```python
from build123d import *

# Parameters (mm, degrees)
SKETCH1_W           = 48
SKETCH1_H           = 5.175
SKETCH1_H_2         = 3
SKETCH1_H_3         = 3.35
BOSS_EXTRUDE1_DEPTH = 2
SKETCH1_3_W         = 48
SKETCH1_3_H         = 3
BOSS_EXTRUDE2_DEPTH = 8.5
CUT_EXTRUDE1_DEPTH  = 27.740991474
CHAMFER1_SIZE       = 0.5


with BuildPart() as part:
    # Sketch1 → Boss-Extrude1 (new body)
    with BuildSketch(Plane.XY):
        with Locations((0, 2.5875)):
            Rectangle(SKETCH1_W, SKETCH1_H)
        with Locations((0, 6.675)):
            Rectangle(SKETCH1_W, SKETCH1_H_2)
        with Locations((0, 9.85)):
            Rectangle(SKETCH1_W, SKETCH1_H_3)
    extrude(amount=BOSS_EXTRUDE1_DEPTH)

    # Sketch1_3 → Boss-Extrude2 (add)
    with BuildSketch(Plane.XY):
        with Locations((0, 6.675)):
            Rectangle(SKETCH1_3_W, SKETCH1_3_H)
    extrude(amount=BOSS_EXTRUDE2_DEPTH)

    # Sketch2 → Cut-Extrude1 (cut, through all)
    with BuildSketch(Plane(origin=(0, 8.175, 0), x_dir=(1, 0, 0), z_dir=(0, 1, 0))):
        with BuildLine():
            Line((-15, -6), (-15, -8.5))
            Line((-15, -8.5), (-10, -8.5))
            Line((-10, -8.5), (-10, -6))
            ThreePointArc((-10, -6), (-12.5, -3.5), (-15, -6))
        make_face()
        with BuildLine():
            Line((10, -8.5), (10, -6))
            ThreePointArc((10, -6), (12.5, -3.5), (15, -6))
            Line((15, -6), (15, -8.5))
            Line((15, -8.5), (10, -8.5))
        make_face()
    extrude(amount=-CUT_EXTRUDE1_DEPTH, mode=Mode.SUBTRACT)

    # Chamfer1
    chamfer1_edges = [part.edges().sort_by_distance(p)[0] for p in [
        (-24, 8.175, 5.25),
        (-24, 5.175, 5.25),
        (24, 5.175, 5.25),
        (24, 8.175, 5.25),
        (-19.5, 8.175, 8.5),
        (-19.5, 5.175, 8.5),
        (0, 5.175, 8.5),
        (19.5, 5.175, 8.5),
        (0, 8.175, 8.5),
        (19.5, 8.175, 8.5),
        (-15, 6.675, 8.5),
        (-10, 6.675, 8.5),
        (15, 6.675, 8.5),
        (10, 6.675, 8.5),
    ]]
    chamfer(chamfer1_edges, length=CHAMFER1_SIZE)


solid = part.part
```
Can you work these out from the model? Positions are in its coordinate system, mm. A direction names the side the tool comes from. Round coordinates to 2 decimals unless told otherwise and drop trailing zeros. Loops run counter-clockwise (first coordinate to the right, second up) from the corner with the lowest first, then second, coordinate; pieces in that order, holes last. Notation, with made-up numbers: M 43,8.5 L 56,8.5 A36 cw 56,46.5 Z; hole C 34,53.25 d9. An arc over 180 degrees is marked long. Answer as a JSON object with one key per item and string values. Group by question number.
Q1. Please list where these lines run through material, in increasing order: L1, parallel to X at y = 6, z = 7.5; L2, parallel to Y at x = 8, z = 5.75 (3 decimals); L3, parallel to Z at x = -2.5, y = 2.5.
Q2. Imagine slicing it at A-A, the plane x = -11. Please give me the cut outline in (y, z) (3 decimals).
Q3. On a 3-axis mill with a long thin cutter (end or side, diameter ignored), from which of +Z, -Z, +X, -X, +Y, -Y can I reach the whole of each face in a straight line? I mean faces 5 (the flat face through (0, 5.175, 5)), 6 (the flat face through (10, 7, 7)), 7 (the flat face through (0, 8.175, 5)). Say none if no direction works.
Q4. Imagine slicing it at C-C, the plane x = 16. Please give me the cut outline in (y, z) (3 decimals), then the cut area to 3 significant figures.
Q5. Will these pins go through, and if not, where does the flat tip stop? pin 1 (1.2 mm diameter, centred on x = -2.5, y = 9, fed in from +Z); pin 2 (3 mm diameter, centred on x = -2, z = 5, fed in from +Y) (3 decimals); pin 3 (1.5 mm diameter, centred on x = -8.5, y = 8.5, fed in from +Z) (3 decimals).
Q6. Imagine slicing it at B-B, the plane z = 5. Please give me the cut outline in (x, y) (3 decimals), then the cut area to 3 significant figures.
Q7. Imagine slicing it at D-D, the plane y = 1. Please give me the cut outline in (x, z).
Q8. We'd pull the mould along X, two halves only. Please class faces 1 (the cylindrical face through (-12.4, 6.7, 3.5)), 2 (the flat face through (0, 2, 2)), 3 (the flat face through (-15, 7, 7)), 4 (the flat face through (24, 6, 2)): +X half, -X half, draft (parallel to the pull), parting line (faces both ways), or undercut.
Findings:
{
 "1": {"L1": "x = -24 to -15, -10 to 10, 15 to 24", "L2": "y = 5.175 to 8.175", "L3": "z = 0 to 2"},
 "2": {"outline": "M 0,0 L 11.525,0 L 11.525,2 L 8.175,2 L 8.175,4 L 5.175,4 L 5.175,2 L 0,2 Z"},
 "3": {"face 5": "+Z, +X, -X, -Y", "face 6": "+Z, +Y, -Y", "face 7": "+Z, +X, -X, +Y"},
 "4": {"outline": "M 0,0 L 11.525,0 L 11.525,2 L 8.175,2 L 8.175,8 L 7.675,8.5 L 5.675,8.5 L 5.175,8 L 5.175,2 L 0,2 Z", "area": "42.3 mm2"},
 "5": {"pin 1": "stops at z = 2", "pin 2": "stops at y = 8.175", "pin 3": "stops at z = 8.425"},
 "6": {"outline": "M -24,5.675 L -23.5,5.175 L -14.791,5.175 L -14.791,8.175 L -23.5,8.175 L -24,7.675 Z; M -10.209,5.175 L 10.209,5.175 L 10.209,8.175 L -10.209,8.175 Z; M 14.791,5.175 L 23.5,5.175 L 24,5.675 L 24,7.675 L 23.5,8.175 L 14.791,8.175 Z", "area": "116 mm2"},
 "7": {"outline": "M -24,0 L 24,0 L 24,2 L -24,2 Z"},
 "8": {"face 1": "undercut", "face 2": "draft", "face 3": "undercut", "face 4": "+X half"}
}
